from build123d import *

# Parameters (mm, degrees)
F0_W     = 50.8
F0_H     = 50.8
F1_DEPTH = 50.8
F4_W     = 19.05
F4_H     = 38.1
F5_DEPTH = 50.8
F7_DEPTH = 76.2


with BuildPart() as f1:
    # F0 (on Front) → F1 (new body)
    with BuildSketch(Plane.XZ):
        Rectangle(F0_W, F0_H)
    extrude(amount=F1_DEPTH)

    # F4 (on offset) → F5 (cut)
    with BuildSketch(Plane.XZ.offset(50.8)):
        with Locations((-15.875, 0)):
            Rectangle(F4_W, F4_H)
        with Locations((15.875, 0)):
            Rectangle(F4_W, F4_H)
    extrude(amount=-F5_DEPTH, mode=Mode.SUBTRACT)

    # F6 (on offset) → F7 (cut)
    with BuildSketch(Plane.XY.offset(50.8)):
        Polygon((-25.4, -6.35), (-25.4, -25.4), (-12.5995083759, -25.4), (-12.5995083759, -38.1), (12.7, -38.1), (12.7, -6.35), align=None)
    extrude(amount=-F7_DEPTH, mode=Mode.SUBTRACT)


solid = f1.part
The listing builds one solid part. Answer for the finished solid, in the listing's coordinates (mm). A direction names the side the tool comes from. Round coordinates to 2 decimals unless told otherwise and drop trailing zeros. Order: outer loops, then holes, each group sorted by start corner. A loop starts at its lowest first (then second) coordinate and runs counter-clockwise, first axis right, second up. Notation, with made-up numbers: (-4.75, 4.25) -> (32.25, 4.25) arc R15 cw to (32.25, 24.25) -> close; hole circle Ø7 at (5.5, -27). An arc over 180 degrees is marked (long way). Write each question's results on one line, items separated by ' | '. Start each with the question number.
Q1. Find section A-A (z = -16). Determine the outline of the cut face in (x, y), then the cut area to 3 significant figures.
Q2. Straight lines are drawn through the part: probe 1 along Z at (x, y) = (-19, -35.5); probe 2 along Y at (x, z) = (-9, -21.5). For each, find the intervals that lie inside material, in ascending order. Write a range as from..to.
Q3. Find section B-B (x = 20). Determine the outline of the cut face in (y, z), then the cut area to 3 significant figures.
Q4. The mould has two halves that part along Z. Classify faces 1 (the flat face through (25.4, -25, -22)), 2 (the flat face through (17, -31, -25.4)), 3 (the flat face through (-18, -38, 19.05)), 4 (the flat face through (-6.35, -3, 0)): pulls with the +Z half, pulls with the -Z half, needs draft (parallel to the pull), parting line crosses it, or undercut.
Q5. Each of these flat-tipped pins is pushed along its axis until it touches: pin 1 (3 mm diameter, centred on y = -2.5, z = -1.5, fed in from +X); pin 2 (3 mm diameter, centred on y = -18, z = -23.5, fed in from -X); pin 3 (10 mm diameter, centred on y = -43.5, z = 2.5, fed in from -X). Where does it stop, or does it pass through?
Q6. Find section C-C (y = -31). Determine the outline of the cut face in (x, z).
Q7. Which of the six approach directions +Z, -Z, +X, -X, +Y, -Y give full straight-line access (tool end or side, diameter ignored) to faces 5 (the flat face through (6.35, -45, 0)), 6 (the flat face through (-6.35, -45, 0)), 7 (the flat face through (-19, -25.4, -22)), 8 (the flat face through (-12.6, -32, -22))?
Q8. Find section D-D (x = -20). Determine the outline of the cut face in (y, z).
Worked answers:
1) outline: (-6.35, -50.8) -> (6.35, -50.8) -> (6.35, -38.1) -> (-6.35, -38.1) -> close; (-6.35, -6.35) -> (6.35, -6.35) -> (6.35, 0) -> (-6.35, 0) -> close | area: 242 mm2
2) probe 1: z = -25.4..-19.05, 19.05..25.4 | probe 2: y = -50.8..-38.1, -6.35..0
3) outline: (-50.8, -25.4) -> (0, -25.4) -> (0, -19.05) -> (-50.8, -19.05) -> close; (-50.8, 19.05) -> (0, 19.05) -> (0, 25.4) -> (-50.8, 25.4) -> close | area: 645 mm2
4) face 1: needs draft | face 2: pulls with the -Z half | face 3: undercut | face 4: undercut
5) pin 1: stops at x = 6.35 | pin 2: stops at x = 12.7 | pin 3: stops at x = -6.35
6) outline: (-25.4, -25.4) -> (-12.6, -25.4) -> (-12.6, -19.05) -> (-25.4, -19.05) -> close; (-25.4, 19.05) -> (-12.6, 19.05) -> (-12.6, 25.4) -> (-25.4, 25.4) -> close; (12.7, -25.4) -> (25.4, -25.4) -> (25.4, -19.05) -> (12.7, -19.05) -> close; (12.7, 19.05) -> (25.4, 19.05) -> (25.4, 25.4) -> (12.7, 25.4) -> close
7) face 5: +X, +Y, -Y | face 6: -X, +Y, -Y | face 7: +Z, -Z, -X | face 8: +Z, -Z
8) outline: (-50.8, -25.4) -> (-25.4, -25.4) -> (-25.4, -19.05) -> (-50.8, -19.05) -> close; (-50.8, 19.05) -> (-25.4, 19.05) -> (-25.4, 25.4) -> (-50.8, 25.4) -> close; (-6.35, -25.4) -> (0, -25.4) -> (0, -19.05) -> (-6.35, -19.05) -> close; (-6.35, 19.05) -> (0, 19.05) -> (0, 25.4) -> (-6.35, 25.4) -> close
